Autodesk Inventor part; units mm, degrees
ref_plane "GIE1_XY" through (0, 0, 0) normal (1, 0, 0) x (0, 0, -1)
ref_plane "GIE1_YZ" through (0, 0, 0) normal (0, 0, -1) x (0, 1, 0)
ref_plane "GIE1_ZX" through (0, 0, 0) normal (0, 1, 0) x (1, 0, 0)
sketch "Skizze_1" plane through (0, 0, 0) normal (0, 0, 1) x (1, 0, 0)
  line L0 (8, 0) -> (0, 0)
  line L1 (0, 0) -> (0, 12)
  line L2 (0, 12) -> (1.3856, 14.4)
  line L3 (1.3856, 14.4) -> (6.6144, 14.4)
  line L4 (6.6144, 14.4) -> (8, 12)
  line L5 (8, 12) -> (8, 0)
  line L6 (8, 0) -> (0, 0)
revolve "Revolution1" add sketch "Skizze_1" angle 360 about axis through (8, 0, 0) along (1, 0, 0)
sketch "Skizze_2_ALT_Drilling_1" plane through (0, 0, 0) normal (0, 0, 1) x (1, 0, 0)
  line L0 (8, 0) -> (0, 0)
  line L1 (0, 0) -> (0, 8)
  line L2 (0, 8) -> (0.8119, 7.1881)
  line L3 (0.8119, 7.1881) -> (7.1881, 7.1881)
  line L4 (7.1881, 7.1881) -> (8, 8)
  line L5 (8, 8) -> (8, 0)
  line L6 (8, 0) -> (0, 0)
revolve "Revolution2" cut sketch "Skizze_2_ALT_Drilling_1" angle 360 about axis through (8, 0, 0) along (1, 0, 0)
sketch "Skizze_3" plane through (0, 0, 0) normal (1, 0, 0) x (0, 1, 0)
  line L0 (-24, 24) -> (-24, -24)
  line L1 (-24, -24) -> (24, -24)
  line L2 (24, -24) -> (24, 24)
  line L3 (24, 24) -> (-24, 24)
  line L4 (-6.9282, 12) -> (-13.8564, 0)
  line L5 (-13.8564, 0) -> (-6.9282, -12)
  line L6 (-6.9282, -12) -> (6.9282, -12)
  line L7 (6.9282, -12) -> (13.8564, 0)
  line L8 (13.8564, 0) -> (6.9282, 12)
  line L9 (6.9282, 12) -> (-6.9282, 12)
extrude "Extrusion1" cut sketch "Skizze_3" along normal blind 8
ref_plane "GIE1_XY" through (0, 0, 0) normal (1, 0, 0) x (0, 0, -1)
ref_plane "GIE1_YZ" through (0, 0, 0) normal (0, 0, -1) x (0, 1, 0)
ref_plane "GIE1_ZX" through (0, 0, 0) normal (0, 1, 0) x (1, 0, 0)
properties part number "V-12-16"
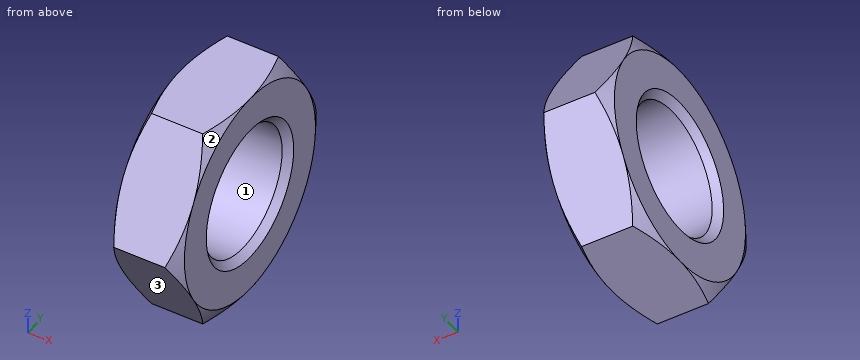
Geometry: final body of the model. Coordinates: model frame, mm. Face numbers are marked on the shaded views. Give positions to 0.01 mm unless a question says otherwise; leave off trailing zeros. Order: outer loops, then holes, each group sorted by start corner. A loop starts at its lowest first (then second) coordinate and runs counter-clockwise, first axis right, second up. Notation, with made-up numbers: M 82,-32 L 98,-32 A12 cw 98,-27 Z; hole C 28,89 d6. An arc over 180 degrees is marked long. Answer as CSV lines item,"result". Start each with the question number.
1) Line query: line 1 (Z direction, x = 4.5, y = 0); line 2 (Z direction, x = 2.75, y = 5.5); line 3 (Y direction, x = 4, z = -3.75). Output: solid intervals per line, ascending. Write a range as from..to.
2) Mould query, pull axis Z, two halves, no side actions, for the marked faces 1, 2 and 3. Classes: +Z half, -Z half, draft (parallel to the pull), parting line (faces both ways), or undercut.
3) Cut plane A-A (x = 4). Output: boundary loops of the cut face in (y, z), then the cut area to 3 significant figures.
4) First-contact query: P1, Ø2, axis at x = 7, z = 3, coming from the -Y side. Flat tip, straight axial feed; report the tip coordinate or a pass-through.
Findings below:
1,line 1,"z = -12..-7.19, 7.19..12"
1,line 2,"z = -12..-4.63, 4.63..12"
1,line 3,"y = -11.69..-6.13, 6.13..11.69"
2,face 1,"undercut"
2,face 2,"+Z half"
2,face 3,"-Z half"
3,outline,"M -13.86,0 L -6.93,-12 L 6.93,-12 L 13.86,0 L 6.93,12 L -6.93,12 Z; hole C 0,0 d14.38"
3,area,"337 mm²"
4,P1,"stops at y = -12.7"
